```python
from build123d import *

# Parameters (mm, degrees)
MAIN_SHAPE_DEPTH                = 6.35
BASE_X_HOLES_D                  = 1.9939
BASE_X_HOLES_DEPTH              = 7.67
BASE_X_HOLES_TIP                = 0.599027994
FILLET1_R                       = 3
SKETCH5_R                       = 3
CUTOUT_FOR_MOUNTING_SCREW_DEPTH = 7.35


with BuildPart() as part:
    # Sketch1 → main shape (new body)
    with BuildSketch(Plane(origin=(0, 0, 0), x_dir=(1, 0, 0), z_dir=(0, 1, 0))):
        Polygon((80, 80), (150, 80), (150, 70), (80, 70), (80, 0), (70, 0), (70, 70), (0, 70), (0, 80), (70, 80), (70, 150), (80, 150), align=None)
    extrude(amount=MAIN_SHAPE_DEPTH)

    # base X holes
    with Locations(Plane(origin=(0, 6.35, 0), x_dir=(-1, 0, 0), z_dir=(0, 1, 0))):
        with Locations((-75, -91), (-59, -75), (-75, -59), (-91, -75)):
            Hole(BASE_X_HOLES_D / 2, depth=BASE_X_HOLES_DEPTH)
            with Locations((0, 0, -(BASE_X_HOLES_DEPTH + BASE_X_HOLES_TIP / 2))):  # 118° drill point
                Cone(0, BASE_X_HOLES_D / 2, BASE_X_HOLES_TIP, mode=Mode.SUBTRACT)

    # Fillet1
    fillet1_edges = [part.edges().sort_by_distance(p)[0] for p in [
        (0, 3.175, -80),
        (70, 3.175, -150),
        (80, 3.175, -150),
        (150, 3.175, -80),
        (150, 3.175, -70),
        (80, 3.175, 0),
        (70, 3.175, 0),
        (0, 3.175, -70),
    ]]
    fillet(fillet1_edges, radius=FILLET1_R)

    # Sketch5 → cutout for mounting screw (cut, through all)
    with BuildSketch(Plane(origin=(0, 0, 0), x_dir=(1, 0, 0), z_dir=(0, 1, 0))):
        with Locations((75, 75)):
            Circle(SKETCH5_R)
    extrude(amount=CUTOUT_FOR_MOUNTING_SCREW_DEPTH, mode=Mode.SUBTRACT)


solid = part.part
```
Design review of the part built by this model. Coordinates are the model's own, in mm. A direction names the side the tool comes from. Give positions to 0.01 mm unless a question says otherwise; leave off trailing zeros. Write each loop counter-clockwise with the first axis right and the second up, starting at its lowest first coordinate (ties: lowest second). Pieces come first, ordered by that corner, then holes. Notation, with made-up numbers: (61, 52) -> (115, 52) arc R29 ccw to (115, 74) -> close; hole circle Ø10 at (73, 17). An arc over 180 degrees is marked (long way). Answer in a Markdown table with one row per item.
(1) For faces 4 (the flat face through (80, 3, -114)), 5 (the flat face through (37, 3, -70)), 6 (the flat face through (80, 3, -37)), 7 (the flat face through (36, 3, -80)), list the 3-axis set-ups (+Z, -Z, +X, -X, +Y, -Y) from which the entire face can be reached by the end or side of a thin tool; tool diameter is ignored.
Results:
| item | result |
|---|---|
| face 4 | -Z, +X, +Y, -Y |
| face 5 | +Z, -X, +Y, -Y |
| face 6 | +Z, +X, +Y, -Y |
| face 7 | -Z, -X, +Y, -Y |
(2) To check wall thickness, follow probe 1 along X at (y, z) = (3.75, -75); probe 2 along Z at (x, y) = (75, 3.25); probe 3 along X at (y, z) = (4, -9). State the ranges of each line that lie inside material, in increasing order.
Results:
| item | result |
|---|---|
| probe 1 | 0 to 58, 60 to 72, 78 to 90, 92 to 150 |
| probe 2 | -150 to -92, -90 to -78, -72 to -60, -58 to 0 |
| probe 3 | 70 to 80 |
(3) Consider section B-B (x = 82.5). State the section outline as (y, z) points.
Results:
| item | result |
|---|---|
| outline | (0, -80) -> (6.35, -80) -> (6.35, -70) -> (0, -70) -> close |
(4) Mouldability with a two-part tool opening along X and no side actions: class faces 1 (the flat face through (114, 3, -70)), 2 (the cylindrical face through (72.6, 3.1, -73.2)), 3 (the flat face through (70, 3, -36)) as +X half, -X half, draft (parallel to the pull), parting line (faces both ways), or undercut.
Results:
| item | result |
|---|---|
| face 1 | draft |
| face 2 | undercut |
| face 3 | -X half |
(5) Consider section A-A (y = 4). State the section outline as (x, z) points.
Results:
| item | result |
|---|---|
| outline | (0, -77) arc R3 ccw to (3, -80) -> (70, -80) -> (70, -147) arc R3 ccw to (73, -150) -> (77, -150) arc R3 ccw to (80, -147) -> (80, -80) -> (147, -80) arc R3 ccw to (150, -77) -> (150, -73) arc R3 ccw to (147, -70) -> (80, -70) -> (80, -3) arc R3 ccw to (77, 0) -> (73, 0) arc R3 ccw to (70, -3) -> (70, -70) -> (3, -70) arc R3 ccw to (0, -73) -> close; hole circle Ø1.99 at (59, -75); hole circle Ø6 at (75, -75); hole circle Ø1.99 at (75, -91); hole circle Ø1.99 at (75, -59); hole circle Ø1.99 at (91, -75) |
(6) Consider section C-C (z = -138). State the section outline as (x, y) points.
Results:
| item | result |
|---|---|
| outline | (70, 0) -> (80, 0) -> (80, 6.35) -> (70, 6.35) -> close |
(7) Clearance check with flat-ended pins moving along their axes: pin 1 (1.5 mm diameter, centred on y = 1, z = -95.5, fed in from -X); pin 2 (1.2 mm diameter, centred on x = 91, z = -75, fed in from +Y); pin 3 (1.9 mm diameter, centred on x = 98.5, y = 2.5, fed in from -Z); pin 4 (1 mm diameter, centred on x = 69, y = 2.5, fed in from +Z). State where each tip first meets the part, or that it passes through.
Results:
| item | result |
|---|---|
| pin 1 | x = 70 |
| pin 2 | through |
| pin 3 | z = -80 |
| pin 4 | z = -70 |
